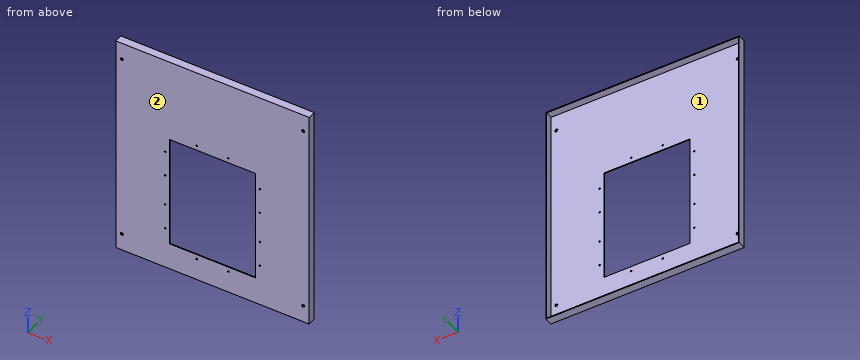
from build123d import *

# Parameters (mm, degrees)
F0_W     = 622.3
F0_H     = 720.725
F0_R     = 4.7625
F0_R_2   = 2.54
F0_W_2   = 278.384
F0_H_2   = 364.236
F1_DEPTH = 25.4
F2_T     = -2.54
F3_W     = 617.22
F3_H     = 22.86
F4_DEPTH = 715.645


with BuildPart() as f1:
    # F0 (on Front) → F1 (new body)
    with BuildSketch(Plane.XZ):
        with Locations((0, 360.3625)):
            Rectangle(F0_W, F0_H)
        with Locations((-292.1, 55.5625)):
            Circle(F0_R, mode=Mode.SUBTRACT)
        with Locations((-50.8, 71.501)):
            Circle(F0_R_2, mode=Mode.SUBTRACT)
        with Locations((-152.654, 135.636)):
            Circle(F0_R_2, mode=Mode.SUBTRACT)
        with Locations((-152.654, 218.186)):
            Circle(F0_R_2, mode=Mode.SUBTRACT)
        with Locations((-152.654, 319.786)):
            Circle(F0_R_2, mode=Mode.SUBTRACT)
        with Locations((50.8, 71.501)):
            Circle(F0_R_2, mode=Mode.SUBTRACT)
        with Locations((152.654, 135.636)):
            Circle(F0_R_2, mode=Mode.SUBTRACT)
        with Locations((292.1, 55.5625)):
            Circle(F0_R, mode=Mode.SUBTRACT)
        with Locations((0, 268.986)):
            Rectangle(F0_W_2, F0_H_2, mode=Mode.SUBTRACT)
        with Locations((152.654, 218.186)):
            Circle(F0_R_2, mode=Mode.SUBTRACT)
        with Locations((152.654, 319.786)):
            Circle(F0_R_2, mode=Mode.SUBTRACT)
        with Locations((-152.654, 402.336)):
            Circle(F0_R_2, mode=Mode.SUBTRACT)
        with Locations((-50.8, 466.471)):
            Circle(F0_R_2, mode=Mode.SUBTRACT)
        with Locations((-292.1, 665.1625)):
            Circle(F0_R, mode=Mode.SUBTRACT)
        with Locations((152.654, 402.336)):
            Circle(F0_R_2, mode=Mode.SUBTRACT)
        with Locations((50.8, 466.471)):
            Circle(F0_R_2, mode=Mode.SUBTRACT)
        with Locations((292.1, 665.1625)):
            Circle(F0_R, mode=Mode.SUBTRACT)
    extrude(amount=F1_DEPTH)

    # F2
    f2_openings = [f1.faces().sort_by_distance(p)[0] for p in [
        (301.627911, 0, 360.3625),
    ]]
    offset(amount=F2_T, openings=f2_openings, kind=Kind.INTERSECTION)

    # F3 (on face) → F4 (cut, through all)
    with BuildSketch(Plane(origin=(0, 0, 718.185), x_dir=(1, 0, 0), z_dir=(0, 0, -1))):
        with Locations((0, 11.43)):
            Rectangle(F3_W, F3_H)
    extrude(amount=F4_DEPTH, mode=Mode.SUBTRACT)


solid = f1.part
The listing builds one solid part. Answer for the finished solid, in the listing's coordinates (mm). Face numbers are marked on the shaded views. Coordinates: 2 decimals unless noted, no trailing zeros. Loops run counter-clockwise (first coordinate to the right, second up) from the corner with the lowest first, then second, coordinate; pieces in that order, holes last.
1) Find section C-C on z = 183.5. Write down the section's boundary in (x, y), then the cut area to 3 significant figures.
2) Flat-ended cylindrical pins translate along their axes: pin 1 Ø8 at (x, z) = (-50.8, 71.501) entering from -Y; pin 2 Ø3 at (x, z) = (-152.654, 135.636) entering from -Y; pin 3 Ø6.5 at (x, z) = (-152.654, 319.786) entering from +Y. Find the tip coordinate at first contact, or state that the pin passes through.
3) Find section D-D on x = -270. Write down the section's boundary in (y, z) (3 decimals), then the cut area to 3 significant figures.
4) Find section B-B on y = -11. Write down the section's boundary in (x, z) (3 decimals), then the cut area to 3 significant figures.
5) Find the intervals of material crossed by L1, parallel to Z at x = -50.8, y = -24.4 (3 decimals); L2, parallel to Z at x = 15, y = -7 (3 decimals); L3, parallel to X at y = -4.25, z = 74.5, in increasing order.
6) Find section A-A on z = 493. Write down the section's boundary in (x, y).
7) Determine the mould class of the marked faces 1 and 2 for opening direction Z: pulls with the +Z half, pulls with the -Z half, needs draft (parallel to the pull), parting line crosses it, or undercut.
Values:
1. outline: (-311.15, -25.4) - (-139.19, -25.4) - (-139.19, -22.86) - (-308.61, -22.86) - (-308.61, 0) - (-311.15, 0) - close; (139.19, -25.4) - (311.15, -25.4) - (311.15, 0) - (308.61, 0) - (308.61, -22.86) - (139.19, -22.86) - close
1. area: 990 mm2
2. pin 1: stops at y = -25.4
2. pin 2: passes through
2. pin 3: stops at y = -22.86
3. outline: (-25.4, 0) - (0, 0) - (0, 2.54) - (-22.86, 2.54) - (-22.86, 718.185) - (0, 718.185) - (0, 720.725) - (-25.4, 720.725) - close
3. area: 1,950 mm2
4. outline: (-311.15, 0) - (311.15, 0) - (311.15, 720.725) - (-311.15, 720.725) - close; hole (-308.61, 2.54) - (308.61, 2.54) - (308.61, 718.185) - (-308.61, 718.185) - close
4. area: 6,800 mm2
5. L1: z = 0 to 68.961, 74.041 to 86.868, 451.104 to 463.931, 469.011 to 720.725
5. L2: z = 0 to 2.54, 718.185 to 720.725
5. L3: x = -311.15 to -308.61, 308.61 to 311.15
6. outline: (-311.15, -25.4) - (311.15, -25.4) - (311.15, 0) - (308.61, 0) - (308.61, -22.86) - (-308.61, -22.86) - (-308.61, 0) - (-311.15, 0) - close
7. face 1: undercut
7. face 2: needs draft
